Model file for the job. Use its own axes, mm. Face numbers are marked on the shaded views. A direction names the side the tool comes from. Round coordinates to 2 decimals unless told otherwise and drop trailing zeros. Loops run counter-clockwise (first coordinate to the right, second up) from the corner with the lowest first, then second, coordinate; pieces in that order, holes last. Notation, with made-up numbers: (83.25, -7) - (115.25, -7) arc R25 ccw to (115.25, 9) - close; hole circle Ø9 at (84, -36). An arc over 180 degrees is marked (long way). Use one line per item in the form item = value.
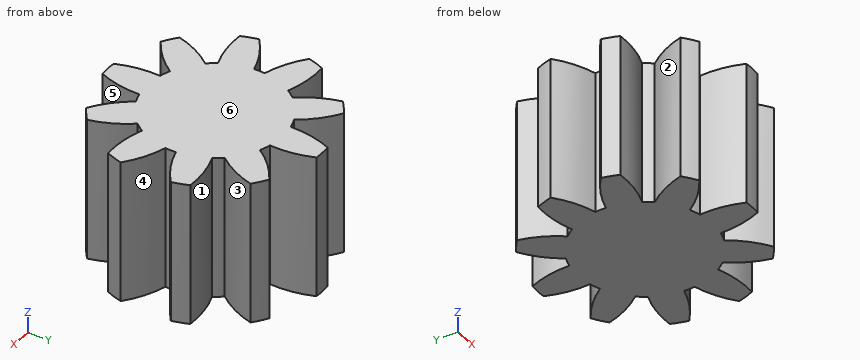
Autodesk Inventor part; units mm, degrees
ref_plane "Work Plane2" through (0, 0, 2) normal (0, 0, 1) x (1, 0, 0)
ref_plane "Work Plane8" through (0, 0, 0) normal (0.9510565, 0.309017, 0) x (0, 0, 1)
ref_plane "Work Plane9" through (0, 0, 0) normal (1, 0, 0) x (0, 1, 0)
sketch "Sketch1" plane through (0, 0, 0) normal (0, 0, 1) x (1, 0, 0)
  circle A0 centre (0, 0) radius 3
  dimension "d0" = 6
extrude "Extrusion1" add sketch "Sketch1" along normal blind 4
ref_plane "Work Plane2" through (0, 0, 2) normal (0, 0, 1) x (1, 0, 0)
sketch "Sketch2" plane through (0, 0, 0) normal (0, 0, -1) x (-1, 0, 0)
  circle A0 centre (0, 0) radius 3
  circle A1 centre (0, 0) radius 2.5
  dimension "d3" = 5
surface extrude "Flankendurchmesser" sketch "Sketch2" against normal through all shown no curves A1
ref_plane "Work Plane8" through (0, 0, 0) normal (0.9510565, 0.309017, 0) x (0, 0, 1)
ref_plane "Work Plane9" through (0, 0, 0) normal (1, 0, 0) x (0, 1, 0)
spur gear teeth "Stirnzahnrad" teeth 10 pitch diameter 5 tip diameter 6 root diameter 3.75 face width 4 start plane through (0, 0, 0) normal (0, 0, -1) x (-1, 0, 0)
equation "\"d0\" = da_da"
equation "\"d1\" = da_b"
equation "\"d3\" = da_dw"
equation "\"d16\" = da_aw"
equation "\"d43\" = da_aw"
equation "\"d46\" = da_aw"
properties part number "Stirnzahnrad1" material "Steel"
1. Cut at A-A, the plane x = -2.6. Give the cut face in (y, z).
Geometry check:
outline = (-1.16, 0) - (-0.47, 0) - (-0.47, 4) - (-1.16, 4) - close; (0.47, 0) - (1.16, 0) - (1.16, 4) - (0.47, 4) - close
2. Flat gauge pin, fed straight in: pin 1 (1 mm diameter, centred on x = -1.5, z = 0.5, fed in from +Y). Where does the tip first touch, or does it go through?
Geometry check:
pin_1 = 2.56
3. Cut at D-D, the plane y = 1.45. Give the cut face in (x, z).
Geometry check:
outline = (-1.59, 0) - (1.59, 0) - (1.59, 4) - (-1.59, 4) - close
4. Tool access for the marked faces 1, 2 and 3: list every direction of +Z, -Z, +X, -X, +Y, -Y with a clear straight run to the whole face (end or side of a thin tool).
Geometry check:
face_1 = +Z, -Z
face_2 = +Z, -Z, -X
face_3 = +Z, -Z, +X
5. Wall check: probe 1 along X at (y, z) = (-1.95, 3); probe 2 along X at (y, z) = (2.5, 3.1); probe 3 along Y at (x, z) = (-0.1, 0.75). Give the ranges that are in metal, low to high.
Geometry check:
probe_1 = -1.85 to -0.88, -0.44 to 0.44, 0.88 to 1.85
probe_2 = -1.66 to -1.48, -0.38 to 0.38, 1.48 to 1.66
probe_3 = -3 to 3
6. Pull direction X, two halves, no side cores. Call the marked faces 4, 5 and 6: +X half, -X half, draft (parallel to the pull), parting line (faces both ways), or undercut.
Geometry check:
face_4 = +X half
face_5 = undercut
face_6 = draft
7. Cut at C-C, the plane x = 2.3. Give the cut face in (y, z), plus the area to 3 significant figures.
Geometry check:
outline = (-1.14, 0) - (-0.31, 0) - (-0.31, 4) - (-1.14, 4) - close; (0.31, 0) - (1.14, 0) - (1.14, 4) - (0.31, 4) - close
area = 6.70 mm^2
8. Cut at B-B, the plane y = -2.4. Give the cut face in (x, z), plus the area to 3 significant figures.
Geometry check:
outline = (-1.8, 0) - (-1.34, 0) - (-1.34, 4) - (-1.8, 4) - close; (-0.4, 0) - (0.4, 0) - (0.4, 4) - (-0.4, 4) - close; (1.34, 0) - (1.8, 0) - (1.8, 4) - (1.34, 4) - close
area = 6.92 mm^2
